Geometry check sheet. Reference: the model listing, model coordinates, mm. Face numbers are marked on the shaded views. A direction names the side the tool comes from. Give positions to 0.01 mm unless a question says otherwise; leave off trailing zeros. Order: outer loops, then holes, each group sorted by start corner. A loop starts at its lowest first (then second) coordinate and runs counter-clockwise, first axis right, second up. Notation, with made-up numbers: M -1,54 L 5,54 A23 ccw 5,92 Z; hole C -7.5,-11 d7. An arc over 180 degrees is marked long. Answer as CSV lines item,"result".
from build123d import *

# Parameters (mm, degrees)
F0_W     = 381
F0_H     = 558.8
F1_DEPTH = 6.35
F2_W     = 381
F2_H     = 6.35
F3_DEPTH = 76.2
F4_W     = 12.7
F4_H     = 533.4
F5_DEPTH = 6.35
F6_W     = 6.35
F6_H     = 533.4
F7_DEPTH = 69.85
F8_W     = 25.4
F8_H     = 57.15
F9_DEPTH = 393.701
F10_R    = 6.35
F12_D    = 6.7564


with BuildPart() as f1:
    # F0 (on Top) → F1 (new body)
    with BuildSketch(Plane.XY):
        Rectangle(F0_W, F0_H)
    extrude(amount=F1_DEPTH)

    # F2 (on face) → F3 (join)
    with BuildSketch(Plane.XY.offset(6.35)):
        with Locations((0, -282.575)):
            Rectangle(F2_W, F2_H)
        with Locations((0, 282.575)):
            Rectangle(F2_W, F2_H)
    extrude(amount=-F3_DEPTH)

    # F4 (on face) → F5 (join)
    with BuildSketch(Plane.XY.offset(6.35)):
        with Locations((196.85, 0)):
            Rectangle(F4_W, F4_H)
    extrude(amount=-F5_DEPTH)

    # F6 (on face) → F7 (join)
    with BuildSketch(Plane(origin=(0, 0, 0), x_dir=(1, 0, 0), z_dir=(0, 0, -1))):
        with Locations((200.025, 0)):
            Rectangle(F6_W, F6_H)
    extrude(amount=F7_DEPTH)

    # F8 (on face) → F9 (cut, through all)
    with BuildSketch(Plane.YZ.offset(203.2)):
        with Locations((0, -41.275)):
            Rectangle(F8_W, F8_H)
    extrude(amount=-F9_DEPTH, mode=Mode.SUBTRACT)

    # F10
    f10_edges = [f1.edges().sort_by_distance(p)[0] for p in [
        (0, 285.75, 6.35),
        (0, -285.75, 6.35),
        (203.2, 0, 6.35),
        (0, -279.4, 0),
        (196.85, 0, 0),
        (0, 279.4, 0),
    ]]
    fillet(f10_edges, radius=F10_R)

    # F12 (through all)
    with Locations(Plane(origin=(0, 0, 0), x_dir=(1, 0, 0), z_dir=(0, 0, -1))):
        with Locations((-171.45, 17.9959), (-171.45, -17.9959)):
            Hole(F12_D / 2)


solid = f1.part
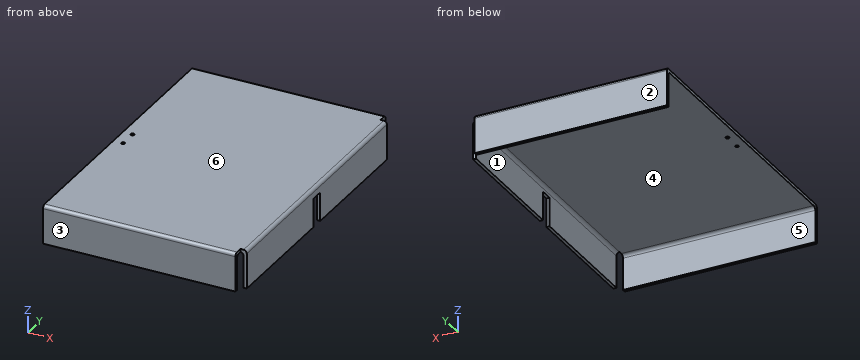
(1) Draft check along Y on the marked faces 3, 4, 5 and 6. Enter one of: +Y half, -Y half, draft (parallel to the pull), parting line (faces both ways), or undercut.
The answers:
face 3,"-Y half"
face 4,"undercut"
face 5,"undercut"
face 6,"draft"
(2) Gauge pin test, flat ends, axial feed: P1, Ø1.5, axis at y = -179, z = -58.5, coming from the -X side; P2, Ø3, axis at x = 199, z = -53, coming from the -Y side; P3, Ø7, axis at x = 198.5, y = 2.5, coming from the -Z side. Record the tip position at first contact, or that the pin passes through.
The answers:
P1,"stops at x = 196.85"
P2,"stops at y = -266.7"
P3,"stops at z = -12.7"
(3) Section check A-A on z = -34. Enter the section's corners in (x, y).
The answers:
outline,"M -190.5,-285.75 L 190.5,-285.75 L 190.5,-279.4 L -190.5,-279.4 Z; M -190.5,279.4 L 190.5,279.4 L 190.5,285.75 L -190.5,285.75 Z; M 196.85,-266.7 L 203.2,-266.7 L 203.2,-12.7 L 196.85,-12.7 Z; M 196.85,12.7 L 203.2,12.7 L 203.2,266.7 L 196.85,266.7 Z"
(4) Section check B-B on x = 3.5. Enter the section's corners in (y, z).
The answers:
outline,"M -285.75,-69.85 L -279.4,-69.85 L -279.4,-6.35 A6.35 cw -273.05,0 L 273.05,0 A6.35 cw 279.4,-6.35 L 279.4,-69.85 L 285.75,-69.85 L 285.75,0 A6.35 ccw 279.4,6.35 L -279.4,6.35 A6.35 ccw -285.75,0 Z"
(5) Material ranges on line 1 (Y direction, x = -171, z = 1); line 2 (Y direction, x = -171, z = 2); line 3 (Y direction, x = -118.5, z = -50), recorded low to high.
The answers:
line 1,"y = -285.67 to -21.34, -14.65 to 14.65, 21.34 to 285.67"
line 2,"y = -285.43 to -21.34, -14.65 to 14.65, 21.34 to 285.43"
line 3,"y = -285.75 to -279.4, 279.4 to 285.75"
(6) Section check C-C on y = 58.5. Enter the section's corners in (x, z), then the cut area to 3 significant figures.
The answers:
outline,"M -190.5,0 L 190.5,0 A6.35 cw 196.85,-6.35 L 196.85,-69.85 L 203.2,-69.85 L 203.2,0 A6.35 ccw 196.85,6.35 L -190.5,6.35 Z"
area,"2,940 mm2"
(7) Tool access check on the marked faces 1 and 2. Record the directions out of +Z, -Z, +X, -X, +Y, -Y that give a thin tool (end or side, any length) a straight path to the whole face; none if there is none.
The answers:
face 1,"-Z, -X, +Y, -Y"
face 2,"+Z, -Z, +X, -X, +Y"
